Verification items for the finished model (mm, model axes). A direction names the side the tool comes from. Give positions to 0.01 mm unless a question says otherwise; leave off trailing zeros. Answer as a JSON object with one key per item and string values.
```python
from build123d import *

# Parameters (mm, degrees)
SKETCH1_W           = 101.6
SKETCH1_H           = 101.6
BOSS_EXTRUDE1_DEPTH = 101.6
SKETCH6_R           = 6.922774564
CUT_EXTRUDE1_DEPTH  = 12.7
CHAMFER2_SIZE       = 2.54


with BuildPart() as part:
    # Sketch1 → Boss-Extrude1 (new body)
    with BuildSketch(Plane.XY):
        with Locations((50.8, 50.8)):
            Rectangle(SKETCH1_W, SKETCH1_H)
    extrude(amount=BOSS_EXTRUDE1_DEPTH)

    # Sketch3 → CSK for 5/16 Flat Head Machine Screw (100)1 (revolve, cut)
    with BuildSketch(Plane(origin=(51.490087233, 83.841482184, 101.6), x_dir=(0, -1, 0), z_dir=(1, 0, 0))):
        Polygon((0, 0), (0, 101.6), (8.0645, 101.6), (4.2164, 98.371060709), (4.2164, 3.228939291), (8.0645, 0), align=None)
    revolve(axis=Axis((51.490087233, 83.841482184, 107.95), (0, 0, -1)), mode=Mode.SUBTRACT)

    # Sketch5 → CBORE for 5/16 Socket Head Cap Screw1 (revolve, cut)
    with BuildSketch(Plane(origin=(101.6, 26.823245181, 55.06253419), x_dir=(0, 0, -1), z_dir=(0, 1, 0))):
        Polygon((0, 0), (0, 101.6), (4.2164, 101.6), (4.2164, 7.9375), (6.74751, 7.9375), (6.74751, 1.105085823), (8.0645, 0), align=None)
    revolve(axis=Axis((107.95, 26.823245181, 55.06253419), (-1, 0, 0)), mode=Mode.SUBTRACT)

    # Sketch6 → Cut-Extrude1 (cut)
    with BuildSketch(Plane.ZY):
        with Locations((55.06253419, 26.823245181)):
            Circle(SKETCH6_R)
    extrude(amount=-CUT_EXTRUDE1_DEPTH, mode=Mode.SUBTRACT)

    # Chamfer2
    chamfer2_edges = [part.edges().sort_by_distance(p)[0] for p in [
        (0, 26.823245181, 48.139759626),
    ]]
    chamfer(chamfer2_edges, length=CHAMFER2_SIZE)


solid = part.part
```
Q1. Section check A-A on x = 54. Count the separate pieces of the cut face and the enclosed holes in it, then the cut area to 3 significant figures.
Resolved:
{"separate pieces": "2", "enclosed holes": "1", "area": "9,550 mm²"}
Q2. Release check for a two-part mould opening along X. For faces 4 (the face through (50.17, 79.64, 3.07)), 5 (the face through (0, 50, 50)), 6 (the face through (50, 52, 101.6)) record: +X half, -X half, draft (parallel to the pull), parting line (faces both ways), or undercut.
Resolved:
{"face 4": "undercut", "face 5": "-X half", "face 6": "draft"}
Q3. Tool access check on faces 1 (the face through (50, 101.6, 50)), 2 (the face through (97.127, 26.527, 61.804)), 3 (the face through (7.55, 31.5, 49.96)). Record the directions out of +Z, -Z, +X, -X, +Y, -Y that give a thin tool (end or side, any length) a straight path to the whole face; none if there is none.
Resolved:
{"face 1": "+Z, -Z, +X, -X, +Y", "face 2": "+X", "face 3": "-X"}
Q4. Gauge pin test, flat ends, axial feed: pin 1 Ø4 at (y, z) = (23, 57.5) entering from -X; pin 2 Ø1 at (y, z) = (35, 54) entering from -X; pin 3 Ø11 at (y, z) = (26.5, 53.5) entering from +X; pin 4 Ø1.5 at (x, y) = (25, 88) entering from -Z. Record the tip position at first contact, or that the pin passes through.
Resolved:
{"pin 1": "stops at x = 12.7", "pin 2": "stops at x = 0.72", "pin 3": "stops at x = 100.79", "pin 4": "stops at z = 0"}
Q5. Material ranges on L1, parallel to Z at x = 71, y = 24; L2, parallel to X at y = 87, z = 92.5; L3, parallel to Y at x = 49.5, z = 70, recorded low to high.
Resolved:
{"L1": "z = 0 to 51.93, 58.19 to 101.6", "L2": "x = 0 to 48.7, 54.28 to 101.6", "L3": "y = 0 to 80.12, 87.56 to 101.6"}
